from build123d import *

# Parameters (mm, degrees)
F0_R     = 10
F1_DEPTH = 50
F2_D     = 20
F2_DEPTH = 51
F2_TIP   = 6.0086061903


# Not quite as in the source:
# - a feature names something its author has since deleted; it is built from what else it names


with BuildPart() as f1:
    # F0 (on Top) → F1 (new body)
    with BuildSketch(Plane.XY):
        with BuildLine():
            Line((0, 19.2077464238), (-13.6434029399, 19.2077464238))
            ThreePointArc((-13.6434029399, 19.2077464238), (-15.252953043, 20.6275337493), (-17.1075657147, 21.7077464238))
            Line((-17.1075657147, 21.7077464238), (0, 21.7077464238))
            Line((0, 21.7077464238), (0, 22.7077464238))
            Line((0, 22.7077464238), (-21.6901414096, 22.7077464238))
            ThreePointArc((-21.6901414096, 22.7077464238), (-26.6650785952, 1.8970379886), (-12.816021735, 18.2077464238))
            Line((-12.816021735, 18.2077464238), (0, 18.2077464238))
            Line((0, 18.2077464238), (0, 19.2077464238))
        make_face()
        with Locations((-21.6901414096, 11.7077464238)):
            Circle(F0_R, mode=Mode.SUBTRACT)
        with Locations((-21.6901414096, 11.7077464238)):
            Circle(F0_R)
    extrude(amount=F1_DEPTH)

    # F2
    with Locations(Plane(origin=(0, 0, 0), x_dir=(1, 0, 0), z_dir=(0, 0, -1))):
        with Locations((-21.6901414096, -11.7077464238)):
            Hole(F2_D / 2, depth=F2_DEPTH)
            with Locations((0, 0, -(F2_DEPTH + F2_TIP / 2))):  # 118° drill point
                Cone(0, F2_D / 2, F2_TIP, mode=Mode.SUBTRACT)


solid = f1.part
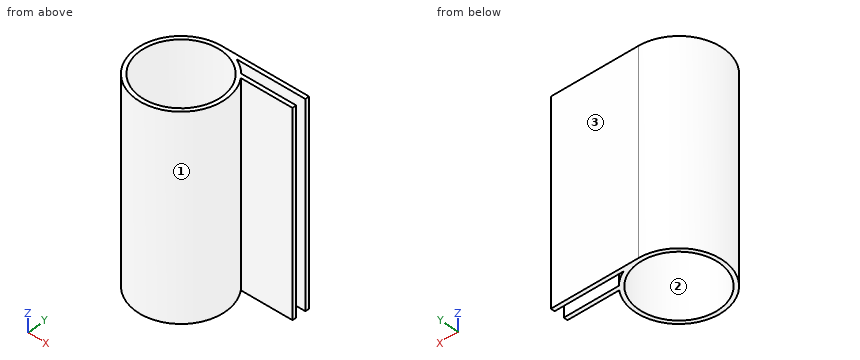
The listing builds one solid part. Answer for the finished solid, in the listing's coordinates (mm). Face numbers are marked on the shaded views. Give positions to 0.01 mm unless a question says otherwise; leave off trailing zeros. Loops run counter-clockwise (first coordinate to the right, second up) from the corner with the lowest first, then second, coordinate; pieces in that order, holes last.
Item 1: A cutting plane is placed at A-A (x = -3). Give the vertices of the cut face in (y, z).
Derived:
outline: (18.21, 0) - (19.21, 0) - (19.21, 50) - (18.21, 50) - close; (21.71, 0) - (22.71, 0) - (22.71, 50) - (21.71, 50) - close
Item 2: Each of these flat-tipped pins is pushed along its axis until it touches: pin 1 Ø4 at (y, z) = (7, 35) entering from -X; pin 2 Ø3 at (x, z) = (-23, 26.5) entering from -Y; pin 3 Ø12 at (x, z) = (-4.5, 37) entering from -Y; pin 4 Ø5 at (x, z) = (-11, 32) entering from -Y. Where does it stop, or does it pass through?
Derived:
pin 1: stops at x = -32.35
pin 2: stops at y = 0.71
pin 3: stops at y = 18.21
pin 4: stops at y = 4.36
Item 3: Determine the mould class of the marked faces 1, 2 and 3 for opening direction X: +X half, -X half, draft (parallel to the pull), parting line (faces both ways), or undercut.
Derived:
face 1: parting line
face 2: undercut
face 3: draft
Item 4: Find the intervals of material crossed by line 1 along Y through (x, z) = (-4.5, 41.5); line 2 along Y through (x, z) = (-15.5, 23); line 3 along X through (y, z) = (16.75, 37.5), in increasing order.
Derived:
line 1: y = 18.21 to 19.21, 21.71 to 22.71
line 2: y = 2.61 to 3.85, 19.56 to 20.8, 21.71 to 22.71
line 3: x = -31.47 to -30.33, -13.05 to -11.91
Item 5: A cutting plane is placed at C-C (z = 43.5). Give the vertices of the cut face in (x, y), then the cut area to 3 significant figures.
Derived:
outline: (-21.69, 22.71) arc R11 ccw (long way) to (-12.82, 18.21) - (0, 18.21) - (0, 19.21) - (-13.64, 19.21) arc R11 ccw to (-17.11, 21.71) - (0, 21.71) - (0, 22.71) - close; hole circle Ø20 at (-21.69, 11.71)
area: 97.8 mm2
Item 6: A cutting plane is placed at B-B (y = 15.5). Give the vertices of the cut face in (x, z).
Derived:
outline: (-32.02, 0) - (-30.94, 0) - (-30.94, 50) - (-32.02, 50) - close; (-12.44, 0) - (-11.36, 0) - (-11.36, 50) - (-12.44, 50) - close
